from build123d import *

# Parameters (mm, degrees)
F0_R     = 1.875
F1_DEPTH = 30
F2_DEPTH = 2
F3_START = 28
F3_DEPTH = 2


with BuildPart() as f1:
    # F0 (on Top) → F1 (new body)
    with BuildSketch(Plane.XY):
        Polygon((16.5, -6.0621778265), (20, 0), (10, 17.3205080757), (3, 17.3205080757), (5, 13.8564064606), (-5, 13.8564064606), (-3, 17.3205080757), (-10, 17.3205080757), (-20, 0), (-16.5, -6.0621778265), (-14.5, -2.5980762114), (-9.5, -11.2583302492), (-13.5, -11.2583302492), (-10, -17.3205080757), (10, -17.3205080757), (13.5, -11.2583302492), (9.5, -11.2583302492), (14.5, -2.5980762114), align=None)
        Circle(F0_R, mode=Mode.SUBTRACT)
    extrude(amount=F1_DEPTH)

    # F0 (on Top) → F2 (join)
    with BuildSketch(Plane.XY):
        Polygon((13.5, -11.2583302492), (16.5, -6.0621778265), (14.5, -2.5980762114), (9.5, -11.2583302492), align=None)
        Polygon((-16.5, -6.0621778265), (-13.5, -11.2583302492), (-9.5, -11.2583302492), (-14.5, -2.5980762114), align=None)
        Polygon((5, 13.8564064606), (3, 17.3205080757), (-3, 17.3205080757), (-5, 13.8564064606), align=None)
    extrude(amount=F2_DEPTH)

    # F0 (on Top) → F3 (join)
    with BuildSketch(Plane.XY.offset(F3_START)):
        Circle(F0_R)
    extrude(amount=F3_DEPTH)


solid = f1.part
Geometry check sheet. Reference: the model listing, model coordinates, mm. A direction names the side the tool comes from. Give positions to 0.01 mm unless a question says otherwise; leave off trailing zeros. Loops run counter-clockwise (first coordinate to the right, second up) from the corner with the lowest first, then second, coordinate; pieces in that order, holes last. Notation, with made-up numbers: (80, 15.5) -> (125, 15.5) arc R16 ccw to (125, 43.5) -> close; hole circle Ø4 at (-20, 10.25). An arc over 180 degrees is marked (long way). Answer in a Markdown table with one row per item. Add a question column.
1) Cross-section at D-D on y = 7. Record the boundary of the cut face in (x, z).
2) Material ranges on probe 1 along Y at (x, z) = (0, 14.75) (1 decimal); probe 2 along Y at (x, z) = (-13, 11); probe 3 along X at (y, z) = (0.5, 24.25), recorded low to high. Write a range as from..to.
3) Cross-section at A-A on x = 0. Record the boundary of the cut face in (y, z) (1 decimal), and give its area (3 significant figures).
4) Set-up check for faces 5 (the face through (-11, -11.258, 16)), 6 (the face through (0, 0, 28)), 7 (the face through (14, -8, 2)), 8 (the face through (12, -11.258, 16)): record each of +Z, -Z, +X, -X, +Y, -Y from which the full face is reachable in a straight line by a thin tool's end or side.
5) Draft check along X on faces 1 (the face through (15.07, 8.54, 14.79)), 2 (the face through (5, 17.321, 15)), 3 (the face through (0, 16, 2)), 4 (the face through (-15.51, -4.35, 15.8)). Enter one of: pulls with the +X half, pulls with the -X half, needs draft (parallel to the pull), parting line crosses it, or undercut.
6) Cross-section at C-C on x = -14. Record the boundary of the cut face in (y, z), and give its area (3 significant figures).
7) Gauge pin test, flat ends, axial feed: P1, Ø7.5, axis at x = 13.5, y = -8.5, coming from the +Z side; P2, Ø1.1, axis at x = -0.5, y = 0, coming from the -Z side; P3, Ø2, axis at y = 1.5, z = 17.5, coming from the -X side; P4, Ø12, axis at y = -5.5, z = 19, coming from the +X side. Record the tip position at first contact, or that the pin passes through.
Outcome:
| question | item | result |
|---|---|---|
| 1 | outline | (-15.96, 0) -> (15.96, 0) -> (15.96, 30) -> (-15.96, 30) -> close |
| 2 | probe 1 | y = -17.3..-1.9, 1.9..13.9 |
| 2 | probe 2 | y = -12.12..-11.26, -5.2..12.12 |
| 2 | probe 3 | x = -19.71..-1.81, 1.81..19.71 |
| 3 | outline | (-17.3, 0) -> (-1.9, 0) -> (-1.9, 28) -> (1.9, 28) -> (1.9, 0) -> (17.3, 0) -> (17.3, 2) -> (13.9, 2) -> (13.9, 30) -> (-17.3, 30) -> close |
| 3 | area | 837 mm^2 |
| 4 | face 5 | +Z, -X |
| 4 | face 6 | -Z |
| 4 | face 7 | +Z |
| 4 | face 8 | +Z, +X |
| 5 | face 1 | pulls with the +X half |
| 5 | face 2 | needs draft |
| 5 | face 3 | undercut |
| 5 | face 4 | undercut |
| 6 | outline | (-10.39, 0) -> (10.39, 0) -> (10.39, 30) -> (-3.46, 30) -> (-3.46, 2) -> (-10.39, 2) -> close |
| 6 | area | 430 mm^2 |
| 7 | P1 | stops at z = 30 |
| 7 | P2 | stops at z = 28 |
| 7 | P3 | stops at x = -19.71 |
| 7 | P4 | stops at x = 20 |
